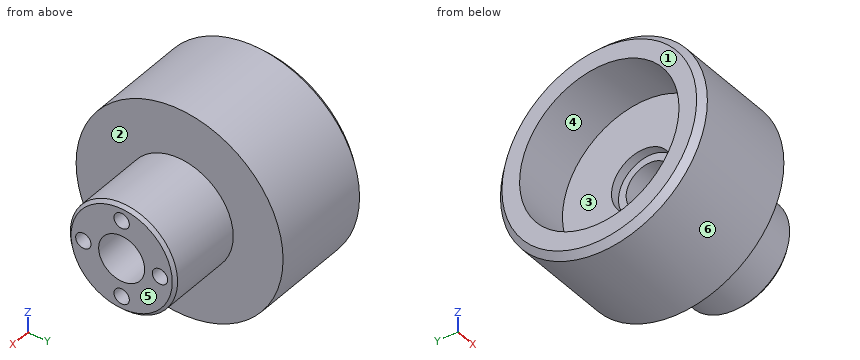
Autodesk Inventor part; units mm, degrees
ref_plane "YZ Plane" through (0, 0, 0) normal (1, 0, 0) x (0, 1, 0)
ref_plane "XZ Plane" through (0, 0, 0) normal (0, 1, 0) x (-1, 0, 0)
ref_plane "XY Plane" through (0, 0, 0) normal (0, 0, 1) x (1, 0, 0)
sketch "Sketch1" plane through (0, 0, 0) normal (0, 0, 1) x (1, 0, 0)
  line L0 (0, 0) -> (0, 33.75)
  line L1 (0, 33.75) -> (35, 33.75)
  line L2 (35, 17.5) -> (60, 17.5)
  line L3 (35, 33.75) -> (35, 17.5)
  line L4 (60, 17.5) -> (60, 0)
  line L5 (0, 0) -> (60, 0)
  dimension "d0" = 33.75
  dimension "d1" = 35
  dimension "d3" = 25
revolve "Revolution1" add sketch "Sketch1" angle 360 about axis through (0, 0, 0) along (1, 0, 0)
thread "Thread1"
sketch "Sketch2" plane through (60, 0, 0) normal (1, 0, 0) x (0, 0, -1)
  circle A0 centre (0, 0) radius 7.5
  dimension "d7" = 15
extrude "Extrusion1" cut sketch "Sketch2" against normal through all
chamfer "Chamfer1" distance 2 angle 45 1 edges at (0, -33.75, 0)
chamfer "Chamfer2" distance 1 angle 45 1 edges at (60, -17.5, 0)
sketch "Sketch3" plane through (0, 0, 0) normal (-1, 0, 0) x (0, 0, 1)
  circle A0 centre (0, 0) radius 26
  dimension "d16" = 52
extrude "Extrusion2" cut sketch "Sketch3" against normal blind 18.5
sketch "Sketch4" plane through (18.5, 0, 0) normal (-1, 0, 0) x (0, 0, 1)
  circle A0 centre (0, 0) radius 10
  dimension "d19" = 20
extrude "Extrusion3" cut sketch "Sketch4" against normal blind 3
sketch "Sketch5" plane through (60, 0, 0) normal (1, 0, 0) x (0, 0, -1)
  circle A0 centre (0, 0) radius 7.5
  circle A1 centre (0, 12.5) radius 2.5
  circle A2 centre (12.5, 0) radius 2.5
  circle A3 centre (0, -12.5) radius 2.5
  circle A4 centre (-12.5, 0) radius 2.5
  dimension "d26" = 5
  dimension "d27" = 5
  dimension "d28" = 5
  dimension "d29" = 5
extrude "Extrusion4" cut sketch "Sketch5" against normal blind 27 contours A1 | A2 | A3 | A4
thread "Thread2"
thread "Thread3"
thread "Thread4"
thread "Thread5"
properties part number "eixo parafuso"
The model under review builds one solid part; all positions refer to its coordinate system, in mm. Face numbers are marked on the shaded views. A direction names the side the tool comes from. Give positions to 0.01 mm unless a question says otherwise; leave off trailing zeros. Write each loop counter-clockwise with the first axis right and the second up, starting at its lowest first coordinate (ties: lowest second). Pieces come first, ordered by that corner, then holes. Notation, with made-up numbers: (-22.75, -19) - (11.25, -19) arc R18 ccw to (11.25, 10) - close; hole circle Ø6 at (-38, 88). An arc over 180 degrees is marked (long way). Answer in a Markdown table with one row per item. Add a question column.
1. Insertion check: P1, Ø6, axis at x = 35.5, z = 13.5, coming from the +Y side; P2, Ø3, axis at x = 45.5, z = 0, coming from the -Y side; P3, Ø6.5, axis at y = 0, z = -12.5, coming from the -X side; P4, Ø5.5, axis at y = 0, z = -12, coming from the +X side. Each pin has a flat end and moves straight along its axis. Give the tip position at first contact, or say it passes through.
2. Draft analysis for pull direction Z (two halves, no side actions). For the marked faces 4, 5 and 6, state which applies: +Z half, -Z half, draft (parallel to the pull), parting line (faces both ways), or undercut.
3. We need section D-D on x = 27. Write out the cut boundary in (y, z).
4. Tool access review of the marked faces 1, 2 and 3: name each direction out of +Z, -Z, +X, -X, +Y, -Y from which nothing blocks a thin tool from reaching the whole face with its end or side.
5. Wall thickness on line 1 along X through (y, z) = (20, 24); line 2 along X through (y, z) = (1, -13); line 3 along Z through (x, y) = (4.5, 18.5): over which ranges is each line inside the solid? List them lowest first. Write a range as [from, to].
6. We need section C-C on x = 56.5. Write out the cut boundary in (y, z).
Ans:
| question | item | result |
|---|---|---|
| 1 | P1 | stops at y = 32.06 |
| 1 | P2 | stops at y = -17.5 |
| 1 | P3 | stops at x = 18.5 |
| 1 | P4 | stops at x = 60 |
| 2 | face 4 | undercut |
| 2 | face 5 | draft |
| 2 | face 6 | parting line |
| 3 | outline | circle Ø67.5 at (0, 0); hole circle Ø15 at (0, 0) |
| 4 | face 1 | +Z, -Z, -X, +Y, -Y |
| 4 | face 2 | +X |
| 4 | face 3 | -X |
| 5 | line 1 | x = [0, 35] |
| 5 | line 2 | x = [18.5, 33] |
| 5 | line 3 | z = [-28.23, -18.27], [18.27, 28.23] |
| 6 | outline | circle Ø35 at (0, 0); hole circle Ø5 at (-12.5, 0); hole circle Ø15 at (0, 0); hole circle Ø5 at (0, -12.5); hole circle Ø5 at (0, 12.5); hole circle Ø5 at (12.5, 0) |
